Geometry: final body of the model. Coordinates: model frame, mm. Give positions to 0.01 mm unless a question says otherwise; leave off trailing zeros. Write each loop counter-clockwise with the first axis right and the second up, starting at its lowest first coordinate (ties: lowest second). Pieces come first, ordered by that corner, then holes. Notation, with made-up numbers: (-11, 61) -> (28, 61) arc R27 ccw to (28, 90) -> close; hole circle Ø11 at (15.5, -32). An arc over 180 degrees is marked (long way). Answer as a JSON object with one key per item and string values. Group by question number.
(1) Material intervals for probe 1 along X at (y, z) = (20, 1.15); probe 2 along X at (y, z) = (13, 1.1); probe 3 along Y at (x, z) = (22, 2.8), sorted ascending.
(2) Draft query along Y for faces 1 (the face through (29, 0, 2)), 2 (the face through (39.5, 26.2, 1.8)), 3 (the face through (-15, 20, 3)), 4 (the face through (31, 40, 2)). Return one class per face: +Y half, -Y half, draft (parallel to the pull), parting line (faces both ways), or undercut.
(3) Section query C-C on z = 1.65. Output: boundary loops of the cut face in (x, y).
(4) Section query D-D on x = 65. Output: boundary loops of the cut face in (y, z).
(5) Section query B-B on x = 22. Output: boundary loops of the cut face in (y, z).
(6) Contact query for flat-ended pins moving along their axis: pin 1 Ø2 at (x, y) = (22, 27) entering from +Z; pin 2 Ø3 at (x, y) = (22.5, 27) entering from +Z; pin 3 Ø5.5 at (x, y) = (22, 13) entering from +Z. Output: stop coordinate, or through.
(7) Section query A-A on y = 27. Output: boundary loops of the cut face in (x, z), plus the area to 3 significant figures.
Autodesk Inventor part; units mm, degrees
ref_plane "YZ Plane" through (0, 0, 0) normal (1, 0, 0) x (0, 1, 0)
ref_plane "XZ Plane" through (0, 0, 0) normal (0, 1, 0) x (-1, 0, 0)
ref_plane "XY Plane" through (0, 0, 0) normal (0, 0, 1) x (1, 0, 0)
sketch "Sketch1" plane through (0, 0, 0) normal (0, 0, 1) x (1, 0, 0)
  line L0 (0, 0) -> (60, 0)
  line L1 (60, 0) -> (60, 40)
  line L2 (60, 40) -> (0, 40)
  line L3 (0, 40) -> (0, 0)
  dimension "d0" = 60
  dimension "d1" = 40
extrude "Extrusion1" add sketch "Sketch1" along normal blind 5
sketch "Sketch6" plane through (0, 0, 5) normal (0, 0, 1) x (1, 0, 0)
  point P0 (0, 0)
  point P1 (30, 20)
hole "Hole2" at (30, 20, 5) direction (0, 0, -1) diameter 11 end through all
sketch "Sketch7" plane through (0, 0, 5) normal (0, 0, 1) x (1, 0, 0)
  line L0 (0, 40) -> (0, 0)
  line L1 (60, 0) -> (60, 40)
  line L2 (60, 0) -> (0, 0)
  line L3 (60, 40) -> (0, 40)
  line L4 (30, 40) -> (30, 0)
  line L5 (0, 0) -> (60, 0)
  line L6 (0, 40) -> (0, 0)
  line L7 (0, 40) -> (-15, 40)
  line L8 (-15, 40) -> (-15, 0)
  line L9 (-15, 0) -> (0, 0)
  line L10 (0, 0) -> (0, 40)
  line L11 (60, 40) -> (60, 0)
  line L12 (60, 40) -> (60, 0)
  line L13 (60, 40) -> (75, 40)
  line L14 (75, 40) -> (75, 0)
  line L15 (75, 0) -> (60, 0)
  line L16 (0, 40) -> (-15, 40)
  point P0 (60, 0)
  point P1 (0, 0)
  dimension "d54" = 15
  dimension "d55" = 40
extrude "Extrusion3" add sketch "Sketch7" against normal blind 5 contours L0 L9 L8 L7 | L13 L14 L15 L1
sketch "Sketch9" plane through (0, 0, 5) normal (0, 0, 1) x (1, 0, 0)
  point P0 (0, 0)
  point P1 (-5, 20)
  point P2 (65, 20)
hole "Hole4" at (-5, 20, 5) at (65, 20, 5) direction (0, 0, -1) diameter 9 end through all
sketch "Sketch10" plane through (0, 0, 5) normal (0, 0, 1) x (1, 0, 0)
  line L0 (35.5, 14.5) -> (35.5, 25.5)
  line L1 (35.5, 14.5) -> (35.5, 25.5)
  line L2 (24.5, 25.5) -> (24.5, 14.5)
  line L3 (24.5, 25.5) -> (24.5, 14.5)
  line L4 (24.5, 14.5) -> (35.5, 25.5) construction
  line L5 (35.5, 14.5) -> (24.5, 25.5) construction
  circle A0 centre (30, 20) radius 5.5
  line L6 (24.5, 30) -> (24.5, 10)
  line L7 (24.5, 10) -> (19.5, 10)
  line L8 (19.5, 10) -> (19.5, 30)
  line L9 (19.5, 30) -> (24.5, 30)
  line L10 (24.5, 20) -> (35.5, 20)
  line L11 (35.5, 30) -> (35.5, 10)
  line L12 (35.5, 10) -> (40.5, 10)
  line L13 (40.5, 10) -> (40.5, 30)
  line L14 (40.5, 30) -> (35.5, 30)
  point P0 (0, 0)
  point P1 (30, 25.5)
  point P2 (22, 13)
  point P3 (22, 27)
  point P4 (38, 13)
  point P5 (38, 27)
  dimension "d45" = 20
  dimension "d46" = 5
hole "Hole5" at (22, 13, 5) at (22, 27, 5) at (38, 13, 5) at (38, 27, 5) direction (0, 0, -1) diameter 3.4 end through all countersink diameter 6.3 countersink angle 90
properties part number "Al block2"
Answer list:
{
 "1": {"probe 1": "-15 to -9.5, -0.5 to 24.5, 35.5 to 60.5, 69.5 to 75", "probe 2": "-15 to 20.3, 23.7 to 36.3, 39.7 to 75", "probe 3": "0 to 11.3, 14.7 to 25.3, 28.7 to 40"},
 "2": {"face 1": "-Y half", "face 2": "undercut", "face 3": "draft", "face 4": "+Y half"},
 "3": {"outline": "(-15, 0) -> (75, 0) -> (75, 40) -> (-15, 40) -> close; hole circle Ø9 at (-5, 20); hole circle Ø3.4 at (22, 13); hole circle Ø3.4 at (22, 27); hole circle Ø11 at (30, 20); hole circle Ø3.4 at (38, 13); hole circle Ø3.4 at (38, 27); hole circle Ø9 at (65, 20)"},
 "4": {"outline": "(0, 0) -> (15.5, 0) -> (15.5, 5) -> (0, 5) -> close; (24.5, 0) -> (40, 0) -> (40, 5) -> (24.5, 5) -> close"},
 "5": {"outline": "(0, 0) -> (11.3, 0) -> (11.3, 3.55) -> (9.85, 5) -> (0, 5) -> close; (14.7, 0) -> (25.3, 0) -> (25.3, 3.55) -> (23.85, 5) -> (16.15, 5) -> (14.7, 3.55) -> close; (28.7, 0) -> (40, 0) -> (40, 5) -> (30.15, 5) -> (28.7, 3.55) -> close"},
 "6": {"pin 1": "through", "pin 2": "z = 3.85", "pin 3": "z = 4.6"},
 "7": {"outline": "(-15, 0) -> (20.3, 0) -> (20.3, 3.55) -> (18.85, 5) -> (-15, 5) -> close; (23.7, 0) -> (36.3, 0) -> (36.3, 3.55) -> (34.85, 5) -> (25.15, 5) -> (23.7, 3.55) -> close; (39.7, 0) -> (75, 0) -> (75, 5) -> (41.15, 5) -> (39.7, 3.55) -> close", "area": "412 mm2"}
}
